Check sheet for the modelled part. Datum: model origin and axes. Units: mm. Coordinates: 2 decimals unless noted, no trailing zeros. Answer as CSV lines item,"result". Start each with the question number.
1) Go/stop test with flat-tipped pins: pin 1 Ø5 at (x, y) = (198.5, 12.5) entering from -Z; pin 2 Ø3.5 at (x, y) = (190.16, 0) entering from -Z; pin 3 Ø1.5 at (y, z) = (-3.5, 5) entering from +X. Record where each tip stops, or that it passes through.
2) Material ranges on L1, parallel to X at y = 1.5, z = 2.5; L2, parallel to X at y = -8, z = 3; L3, parallel to X at y = -11.5, z = 1.25, recorded low to high. Write a range as [from, to].
3) Draft check along X on faces 1 (the cylindrical face through (-92.415, 9.665, 3.131)), 2 (the cylindrical face through (-108.29, -0.42, 3.13)), 3 (the cylindrical face through (234.602, 0.419, 3.131)). Enter one of: +X half, -X half, draft (parallel to the pull), parting line (faces both ways), or undercut.
4) Section check A-A (z = 4). State how many separate pieces and enclosed holes the cut face has, and give its area (3 significant figures).
from build123d import *

# Parameters (mm, degrees)
SKETCH1_R           = 3.175
SKETCH1_R_2         = 2.1828125
BOSS_EXTRUDE1_DEPTH = 6.35


with BuildPart() as part:
    # Sketch1 → Boss-Extrude1 (new body)
    with BuildSketch(Plane.XY):
        with BuildLine():
            Line((-89.243243243, 19.05), (215.556756757, 19.05))
            ThreePointArc((215.556756757, 19.05), (234.606756757, 0), (215.556756757, -19.05))
            Line((215.556756757, -19.05), (-89.243243243, -19.05))
            ThreePointArc((-89.243243243, -19.05), (-108.293243243, 0), (-89.243243243, 19.05))
        make_face()
        with Locations((63.156756757, 0)):
            Circle(SKETCH1_R, mode=Mode.SUBTRACT)
        with Locations((-0.343243243, 0)):
            Circle(SKETCH1_R_2, mode=Mode.SUBTRACT)
        with Locations((126.656756757, 0)):
            Circle(SKETCH1_R_2, mode=Mode.SUBTRACT)
        with Locations((215.556756757, -9.525)):
            Circle(SKETCH1_R, mode=Mode.SUBTRACT)
        with Locations((215.556756757, 9.525)):
            Circle(SKETCH1_R, mode=Mode.SUBTRACT)
        with Locations((-89.243243243, 9.525)):
            Circle(SKETCH1_R, mode=Mode.SUBTRACT)
        with Locations((-89.243243243, -9.525)):
            Circle(SKETCH1_R, mode=Mode.SUBTRACT)
        with Locations((-63.843243243, 0)):
            Circle(SKETCH1_R_2, mode=Mode.SUBTRACT)
        with Locations((190.156756757, 0)):
            Circle(SKETCH1_R_2, mode=Mode.SUBTRACT)
    extrude(amount=BOSS_EXTRUDE1_DEPTH)


solid = part.part
Results found:
1,pin 1,"stops at z = 0"
1,pin 2,"passes through"
1,pin 3,"stops at x = 234.41"
2,L1,"x = [-108.23, -65.43], [-62.26, -1.93], [1.24, 60.36], [65.96, 125.07], [128.24, 188.57], [191.74, 234.55]"
2,L2,"x = [-106.53, -92.03], [-86.46, 212.77], [218.34, 232.85]"
2,L3,"x = [-104.43, -91.73], [-86.76, 213.07], [218.04, 230.74]"
3,face 1,"undercut"
3,face 2,"-X half"
3,face 3,"+X half"
4,separate pieces,"1"
4,enclosed holes,"9"
4,area,"12,500 mm2"
